Verification items for the finished model (mm, model axes). A direction names the side the tool comes from. Give positions to 0.01 mm unless a question says otherwise; leave off trailing zeros. Loops run counter-clockwise (first coordinate to the right, second up) from the corner with the lowest first, then second, coordinate; pieces in that order, holes last. Notation, with made-up numbers: M 37.25,76 L 80.25,76 A17 cw 80.25,88 Z; hole C 45,85.25 d5. An arc over 180 degrees is marked long. Use a Markdown table: item, result.
from build123d import *

# Parameters (mm, degrees)
F2_DEPTH    = 2.5
F3_DEPTH    = 10
F4_DEPTH    = 3
F5_DEPTH    = 6
F6_T1_DEPTH = 5
F8_DEPTH    = 14
F9_DEPTH    = 9
F10_DEPTH   = 1
F11_DEPTH   = 16.5
F13_DEPTH   = 6
F14_R       = 2.49999


# Not quite as in the source:
# - a fillet or chamfer that OpenCascade refuses, or shapes differently, is made with other operations: its cross-section is extruded or revolved along the edge and cut away or added
# - a fillet or chamfer is up to 0.001 mm smaller than in the source, because OpenCascade refuses the exact size


with BuildPart() as f2:
    # F0 (on Front) → F2 (new body, symmetric)
    with BuildSketch(Plane.XZ):
        Polygon((0, 3.5), (0, 0), (9, 0), (9, 14), (6, 14), (6, 3.5), align=None)
    extrude(amount=F2_DEPTH, both=True)

    # F1 (on Right) → F3 (join)
    with BuildSketch(Plane.YZ):
        with BuildLine():
            Line((-2.5, 14), (2.5, 14))
            ThreePointArc((2.5, 14), (0, 16.5), (-2.5, 14))
        make_face()
        with BuildLine():
            ThreePointArc((-2.5, 14), (0, 11.5), (2.5, 14))
            Line((2.5, 14), (-2.5, 14))
        make_face()
    extrude(amount=F3_DEPTH)

    # F1 (on Right) → F4 (cut)
    with BuildSketch(Plane.YZ):
        with BuildLine():
            Line((-2.5, 14), (2.5, 14))
            ThreePointArc((2.5, 14), (0, 16.5), (-2.5, 14))
        make_face()
        with BuildLine():
            ThreePointArc((-2.5, 14), (0, 11.5), (2.5, 14))
            Line((2.5, 14), (-2.5, 14))
        make_face()
    extrude(amount=F4_DEPTH, mode=Mode.SUBTRACT)

    # F1 (on Right) → F5 (cut)
    with BuildSketch(Plane.YZ):
        with BuildLine():
            ThreePointArc((-2.5, 14), (0, 11.5), (2.5, 14))
            Line((2.5, 14), (-2.5, 14))
        make_face()
    extrude(amount=F5_DEPTH, mode=Mode.SUBTRACT)

    # F6: fillet of radius 1 on 2 edges, made by hand

    # F6_s2 → F6_t1 (join)
    with BuildSketch(Plane.XZ.offset(-2.5)):
        with BuildLine():
            ThreePointArc((6, 13), (5.7071067812, 13.7071067812), (5, 14))
            Line((5, 14), (6, 14))
            Line((6, 14), (6, 13))
        make_face()
        with BuildLine():
            ThreePointArc((5, 3.5), (5.7071067812, 3.7928932188), (6, 4.5))
            Line((6, 4.5), (6, 3.5))
            Line((6, 3.5), (5, 3.5))
        make_face()
    extrude(amount=F6_T1_DEPTH)

    # F7 (on Top) → F8 (join)
    with BuildSketch(Plane.XY):
        Polygon((9, 2.5), (9, -2.5), (10, 0), align=None)
    extrude(amount=F8_DEPTH)

    # F7 (on Top) → F9 (cut)
    with BuildSketch(Plane.XY):
        Polygon((9, 2.5), (9, -2.5), (10, 0), align=None)
    extrude(amount=F9_DEPTH, mode=Mode.SUBTRACT)

    # F10 (add): a face of the model
    f10_faces = [f2.faces().sort_by_distance(p)[0] for p in [
        (10, -1.717766953, 12.282233047),
    ]]
    extrude(f10_faces, amount=F10_DEPTH)

    # F7 (on Top) → F11 (cut)
    with BuildSketch(Plane.XY):
        Polygon((11, 0), (10, -2.5), (11.5, -2.5), (11.5, 2.5), (10, 2.5), align=None)
    extrude(amount=F11_DEPTH, mode=Mode.SUBTRACT)

    # F12: F2 across face


with BuildPart() as f2_1:
    add(f2.part)
    add(f2.part.mirror(Plane(origin=(0, 0, 1.75), x_dir=(0, -1, 0), z_dir=(-1, 0, 0))))

    # F13 (add): a face of the model
    f13_faces = [f2_1.faces().sort_by_distance(p)[0] for p in [
        (0, 0, 0),
    ]]
    extrude(f13_faces, amount=F13_DEPTH)

    # F14 (radius 2.5 in the source; OpenCascade refuses exactly that, so slightly less here)
    f14_edges = [f2_1.edges().sort_by_distance(p)[0] for p in [
        (0, -2.5, -6),
        (0, 2.5, -6),
    ]]
    fillet(f14_edges, radius=F14_R)


solid = f2_1.part
(1) Cross-section at D-D on z = 7. Record the cut outline in (x, y).
Results below:
| item | result |
|---|---|
| outline | M -9,-2.5 L -6,-2.5 L -6,2.5 L -9,2.5 Z; M 6,-2.5 L 9,-2.5 L 9,2.5 L 6,2.5 Z |
(2) Cross-section at A-A on z = 10. Record the cut outline in (x, y).
Results below:
| item | result |
|---|---|
| outline | M -10,0 L -9,-2.5 L -6,-2.5 L -6,2.5 L -9,2.5 Z; M 6,-2.5 L 9,-2.5 L 10,0 L 9,2.5 L 6,2.5 Z |
(3) Draft check along Z on faces 5 (the cylindrical face through (-6.94, 0.54, 16.44)), 6 (the cylindrical face through (0, 2, -5)), 7 (the cylindrical face through (-5.699, 0.035, 3.785)), 8 (the flat face through (9, 0, 2)). Enter one of: +Z half, -Z half, draft (parallel to the pull), parting line (faces both ways), or undercut.
Results below:
| item | result |
|---|---|
| face 5 | parting line |
| face 6 | -Z half |
| face 7 | undercut |
| face 8 | draft |
(4) Material ranges on line 1 (X direction, y = -1.05, z = 8.25); line 2 (Z direction, x = -3.25, y = -0.1); line 3 (X direction, y = -0.2, z = -1.5), recorded low to high.
Results below:
| item | result |
|---|---|
| line 1 | -9 to -6, 6 to 9 |
| line 2 | -6 to 3.5, 14 to 16.5 |
| line 3 | -9 to 9 |
(5) Gauge pin test, flat ends, axial feed: P1, Ø0.5, axis at x = -9.5, y = 0, coming from the -Z side; P2, Ø1, axis at x = -6, y = 1.5, coming from the -Z side; P3, Ø2.5, axis at y = 0.5, z = 7.5, coming from the -X side. Record the tip position at first contact, or that the pin passes through.
Results below:
| item | result |
|---|---|
| P1 | z = 9 |
| P2 | z = -5.79 |
| P3 | x = -9 |
(6) Set-up check for faces 1 (the flat face through (-9.49, -1.27, 10.35)), 2 (the flat face through (9.4, 0, 9)), 3 (the cylindrical face through (5.699, 0.035, 3.785)), 4 (the flat face through (9.51, 1.23, 10.35)): record each of +Z, -Z, +X, -X, +Y, -Y from which the full face is reachable in a straight line by a thin tool's end or side.
Results below:
| item | result |
|---|---|
| face 1 | -Z, -X, -Y |
| face 2 | -Z, +X, +Y, -Y |
| face 3 | +Y, -Y |
| face 4 | -Z, +X, +Y |
(7) Cross-section at C-C on y = 1.35. Record the cut outline in (x, z), then the cut area to 3 significant figures.
Results below:
| item | result |
|---|---|
| outline | M -10.46,11.9 L -9.46,11.9 L -9.46,9 L -9,9 L -9,-5.6 L 9,-5.6 L 9,9 L 9.46,9 L 9.46,11.9 L 10.46,11.9 L 10.46,16.1 L 3,16.1 L 3,14 L 5,14 A1 cw 6,13 L 6,4.5 A1 cw 5,3.5 L -5,3.5 A1 cw -6,4.5 L -6,13 A1 cw -5,14 L -3,14 L -3,16.1 L -10.46,16.1 Z |
| area | 268 mm^2 |
